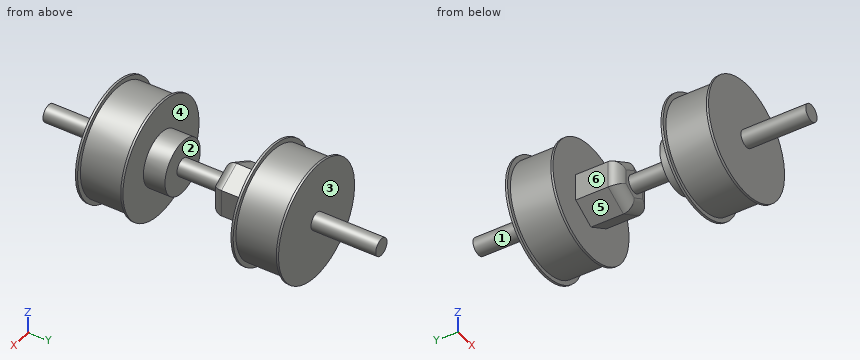
```python
from build123d import *

# Parameters (mm, degrees)
SKETCH2_R            = 27
BOSS_EXTRUDE1_DEPTH  = 1
SKETCH3_R            = 12.5
BOSS_EXTRUDE2_DEPTH  = 10
SKETCH4_R            = 4
BOSS_EXTRUDE3_DEPTH  = 20
BOSS_EXTRUDE4_DEPTH  = 20
FILLET1_R            = 5
SKETCH6_R            = 27
BOSS_EXTRUDE5_DEPTH  = 1
SKETCH7_R            = 25
BOSS_EXTRUDE6_DEPTH  = 20
SKETCH8_R            = 27
BOSS_EXTRUDE7_DEPTH  = 1
SKETCH9_R            = 4
BOSS_EXTRUDE8_DEPTH  = 30
SKETCH10_R           = 25
BOSS_EXTRUDE9_DEPTH  = 20
SKETCH11_R           = 27
BOSS_EXTRUDE10_DEPTH = 1
SKETCH12_R           = 4
BOSS_EXTRUDE11_DEPTH = 30


with BuildPart() as part:
    # Sketch2 → Boss-Extrude1 (new body)
    with BuildSketch(Plane(origin=(0, 0, 0), x_dir=(1, 0, 0), z_dir=(0, 1, 0))):
        Circle(SKETCH2_R)
    extrude(amount=BOSS_EXTRUDE1_DEPTH)

    # Sketch3 → Boss-Extrude2 (add)
    with BuildSketch(Plane(origin=(0, 1, 0), x_dir=(1, 0, 0), z_dir=(0, 1, 0))):
        Circle(SKETCH3_R)
    extrude(amount=BOSS_EXTRUDE2_DEPTH)

    # Sketch4 → Boss-Extrude3 (add)
    with BuildSketch(Plane(origin=(0, 11, 0), x_dir=(1, 0, 0), z_dir=(0, 1, 0))):
        Circle(SKETCH4_R)
    extrude(amount=BOSS_EXTRUDE3_DEPTH)

    # Sketch5 → Boss-Extrude4 (add)
    with BuildSketch(Plane(origin=(0, 31, 0), x_dir=(1, 0, 0), z_dir=(0, 1, 0))):
        Polygon((0, 12.5), (10.825317547, 6.25), (10.825317547, -6.25), (0, -12.5), (-10.825317547, -6.25), (-10.825317547, 6.25), align=None)
    extrude(amount=BOSS_EXTRUDE4_DEPTH)

    # Fillet1
    fillet1_edges = [part.edges().sort_by_distance(p)[0] for p in [
        (-5.412658774, 31, -9.375),
        (-10.825317547, 31, 0),
        (-5.412658774, 31, 9.375),
        (5.412658774, 31, 9.375),
        (10.825317547, 31, 0),
        (5.412658774, 31, -9.375),
    ]]
    fillet(fillet1_edges, radius=FILLET1_R)

    # Sketch6 → Boss-Extrude5 (add)
    with BuildSketch(Plane(origin=(0, 51, 0), x_dir=(1, 0, 0), z_dir=(0, 1, 0))):
        Circle(SKETCH6_R)
    extrude(amount=BOSS_EXTRUDE5_DEPTH)

    # Sketch7 → Boss-Extrude6 (add)
    with BuildSketch(Plane(origin=(0, 52, 0), x_dir=(1, 0, 0), z_dir=(0, 1, 0))):
        Circle(SKETCH7_R)
    extrude(amount=BOSS_EXTRUDE6_DEPTH)

    # Sketch8 → Boss-Extrude7 (add)
    with BuildSketch(Plane(origin=(0, 72, 0), x_dir=(1, 0, 0), z_dir=(0, 1, 0))):
        Circle(SKETCH8_R)
    extrude(amount=BOSS_EXTRUDE7_DEPTH)

    # Sketch9 → Boss-Extrude8 (add)
    with BuildSketch(Plane(origin=(0, 73, 0), x_dir=(1, 0, 0), z_dir=(0, 1, 0))):
        Circle(SKETCH9_R)
    extrude(amount=BOSS_EXTRUDE8_DEPTH)

    # Sketch10 → Boss-Extrude9 (add)
    with BuildSketch(Plane(origin=(0, 0, 0), x_dir=(-1, 0, 0), z_dir=(0, -1, 0))):
        Circle(SKETCH10_R)
    extrude(amount=BOSS_EXTRUDE9_DEPTH)

    # Sketch11 → Boss-Extrude10 (add)
    with BuildSketch(Plane(origin=(0, -20, 0), x_dir=(-1, 0, 0), z_dir=(0, -1, 0))):
        Circle(SKETCH11_R)
    extrude(amount=BOSS_EXTRUDE10_DEPTH)

    # Sketch12 → Boss-Extrude11 (add)
    with BuildSketch(Plane(origin=(0, -21, 0), x_dir=(-1, 0, 0), z_dir=(0, -1, 0))):
        Circle(SKETCH12_R)
    extrude(amount=BOSS_EXTRUDE11_DEPTH)


solid = part.part
```
The listing builds one solid part. Answer for the finished solid, in the listing's coordinates (mm). Face numbers are marked on the shaded views. A direction names the side the tool comes from. Round coordinates to 2 decimals unless told otherwise and drop trailing zeros. Order: outer loops, then holes, each group sorted by start corner. A loop starts at its lowest first (then second) coordinate and runs counter-clockwise, first axis right, second up. Notation, with made-up numbers: (76, 19) -> (119, 19) arc R21 ccw to (119, 57) -> close; hole circle Ø10 at (24.5, -26.75). An arc over 180 degrees is marked (long way). Answer as CSV lines item,"result".
Q1. A cutting plane is placed at D-D on y = 3.5. Determine the outline of the cut face in (x, z).
Computed values:
outline,"circle Ø25 at (0, 0)"
Q2. Given pin 1 (6 mm diameter, centred on x = 16, z = -6.5, fed in from +Y); pin 2 (6 mm diameter, centred on y = 33, z = 18, fed in from +X); pin 3 (1 mm diameter, centred on y = 62.5, z = 16.5, fed in from -X); pin 4 (10 mm diameter, centred on y = 43, z = 1, fed in from +X), each flat-ended and moving along its own axis, determine where each tip first touches the part or whether it passes through.
Computed values:
pin 1,"stops at y = 73"
pin 2,"passes through"
pin 3,"stops at x = -19.21"
pin 4,"stops at x = 10.83"
Q3. For a pull along Y with two mould halves and no side action, classify the marked faces 1, 2 and 3 as +Y half, -Y half, draft (parallel to the pull), parting line (faces both ways), or undercut.
Computed values:
face 1,"draft"
face 2,"undercut"
face 3,"+Y half"
Q4. A cutting plane is placed at C-C on y = 49.5. Determine the outline of the cut face in (x, z).
Computed values:
outline,"(-10.83, -6.25) -> (0, -12.5) -> (10.83, -6.25) -> (10.83, 6.25) -> (0, 12.5) -> (-10.83, 6.25) -> close"
Q5. Consider line 1 (Y direction, x = -22, z = -15); line 2 (Y direction, x = -16, z = 14); line 3 (X direction, y = -9, z = 0). Determine where each line is inside the solid, lowest interval first. Write a range as from..to.
Computed values:
line 1,"y = -21..-20, 0..1, 51..52, 72..73"
line 2,"y = -21..1, 51..73"
line 3,"x = -25..25"
Q6. A cutting plane is placed at A-A on z = 18. Determine the outline of the cut face in (x, y), plus the area to 3 significant figures.
Computed values:
outline,"(-20.12, -21) -> (20.12, -21) -> (20.12, -20) -> (17.35, -20) -> (17.35, 0) -> (20.12, 0) -> (20.12, 1) -> (-20.12, 1) -> (-20.12, 0) -> (-17.35, 0) -> (-17.35, -20) -> (-20.12, -20) -> close; (-20.12, 51) -> (20.12, 51) -> (20.12, 52) -> (17.35, 52) -> (17.35, 72) -> (20.12, 72) -> (20.12, 73) -> (-20.12, 73) -> (-20.12, 72) -> (-17.35, 72) -> (-17.35, 52) -> (-20.12, 52) -> close"
area,"1,550 mm^2"
Q7. A cutting plane is placed at B-B on x = 18.5. Determine the outline of the cut face in (y, z).
Computed values:
outline,"(-21, -19.67) -> (-20, -19.67) -> (-20, -16.82) -> (0, -16.82) -> (0, -19.67) -> (1, -19.67) -> (1, 19.67) -> (0, 19.67) -> (0, 16.82) -> (-20, 16.82) -> (-20, 19.67) -> (-21, 19.67) -> close; (51, -19.67) -> (52, -19.67) -> (52, -16.82) -> (72, -16.82) -> (72, -19.67) -> (73, -19.67) -> (73, 19.67) -> (72, 19.67) -> (72, 16.82) -> (52, 16.82) -> (52, 19.67) -> (51, 19.67) -> close"
Q8. Which of the six approach directions +Z, -Z, +X, -X, +Y, -Y give full straight-line access (tool end or side, diameter ignored) to the marked faces 4, 5 and 6?
Computed values:
face 4,"none"
face 5,"-Z, -X"
face 6,"+Z, -Z, -X"
